from build123d import *

# Parameters (mm, degrees)
SKETCH_1_W          = 32
SKETCH_1_H          = 32
EXTRUDE_1_DEPTH     = 8
CUT_EXTRUDE_1_REACH = 10
SKETCH_2_R          = 1.5
SKETCH_3_R          = 13.25
CUT_EXTRUDE_2_DEPTH = 2.2
SKETCH_4_R          = 5.1
CUT_EXTRUDE_3_DEPTH = 3.5
CUT_EXTRUDE_4_REACH = 4.3
SKETCH_5_R          = 3
FILLET_1_R          = 2


with BuildPart() as part:
    # 草图1 → 凸台-拉伸1 (new body)
    with BuildSketch(Plane.XY):
        Rectangle(SKETCH_1_W, SKETCH_1_H)
    extrude(amount=EXTRUDE_1_DEPTH)

    # 草图2 → 切除-拉伸1 (cut, up to next)
    with BuildSketch(Plane.XY.offset(8), mode=Mode.PRIVATE) as cut_extrude_1_sk1:
        with Locations((-13.258252147, 13.258252147)):
            Circle(SKETCH_2_R)
    cut_extrude_1_tool1 = extrude(cut_extrude_1_sk1.sketch, amount=-CUT_EXTRUDE_1_REACH, mode=Mode.PRIVATE) & part.part
    add(cut_extrude_1_tool1.solids().sort_by_distance((-13.258252, 13.258252, 8))[0], mode=Mode.SUBTRACT)
    # 草图2 → 切除-拉伸1 (cut, up to next)
    with BuildSketch(Plane.XY.offset(8), mode=Mode.PRIVATE) as cut_extrude_1_sk2:
        with Locations((13.258252147, 13.258252147)):
            Circle(SKETCH_2_R)
    cut_extrude_1_tool2 = extrude(cut_extrude_1_sk2.sketch, amount=-CUT_EXTRUDE_1_REACH, mode=Mode.PRIVATE) & part.part
    add(cut_extrude_1_tool2.solids().sort_by_distance((13.258252, 13.258252, 8))[0], mode=Mode.SUBTRACT)
    # 草图2 → 切除-拉伸1 (cut, up to next)
    with BuildSketch(Plane.XY.offset(8), mode=Mode.PRIVATE) as cut_extrude_1_sk3:
        with Locations((13.258252147, -13.258252147)):
            Circle(SKETCH_2_R)
    cut_extrude_1_tool3 = extrude(cut_extrude_1_sk3.sketch, amount=-CUT_EXTRUDE_1_REACH, mode=Mode.PRIVATE) & part.part
    add(cut_extrude_1_tool3.solids().sort_by_distance((13.258252, -13.258252, 8))[0], mode=Mode.SUBTRACT)
    # 草图2 → 切除-拉伸1 (cut, up to next)
    with BuildSketch(Plane.XY.offset(8), mode=Mode.PRIVATE) as cut_extrude_1_sk4:
        with Locations((-13.258252147, -13.258252147)):
            Circle(SKETCH_2_R)
    cut_extrude_1_tool4 = extrude(cut_extrude_1_sk4.sketch, amount=-CUT_EXTRUDE_1_REACH, mode=Mode.PRIVATE) & part.part
    add(cut_extrude_1_tool4.solids().sort_by_distance((-13.258252, -13.258252, 8))[0], mode=Mode.SUBTRACT)

    # 草图3 → 切除-拉伸2 (cut)
    with BuildSketch(Plane.XY.offset(8)):
        Circle(SKETCH_3_R)
    extrude(amount=-CUT_EXTRUDE_2_DEPTH, mode=Mode.SUBTRACT)

    # 草图4 → 切除-拉伸3 (cut)
    with BuildSketch(Plane.XY.offset(5.8)):
        Circle(SKETCH_4_R)
    extrude(amount=-CUT_EXTRUDE_3_DEPTH, mode=Mode.SUBTRACT)

    # 草图5 → 切除-拉伸4 (cut, up to next)
    with BuildSketch(Plane.XY.offset(2.3), mode=Mode.PRIVATE) as cut_extrude_4_sk1:
        Circle(SKETCH_5_R)
    cut_extrude_4_tool1 = extrude(cut_extrude_4_sk1.sketch, amount=-CUT_EXTRUDE_4_REACH, mode=Mode.PRIVATE) & part.part
    add(cut_extrude_4_tool1.solids().sort_by_distance((0, 0, 2.3))[0], mode=Mode.SUBTRACT)

    # 圆角1
    fillet_1_edges = [part.edges().sort_by_distance(p)[0] for p in [
        (16, -16, 4),
        (-16, -16, 4),
        (-16, 16, 4),
        (16, 16, 4),
    ]]
    fillet(fillet_1_edges, radius=FILLET_1_R)


solid = part.part
For this review, take the finished solid that the model builds, in its own axes (mm). A direction names the side the tool comes from. Give positions to 0.01 mm unless a question says otherwise; leave off trailing zeros. Loops run counter-clockwise (first coordinate to the right, second up) from the corner with the lowest first, then second, coordinate; pieces in that order, holes last.
Item 1: Draft analysis for pull direction X (two halves, no side actions). For faces 1 (the cylindrical face through (-14.757, -13.192, 4.056)), 2 (the cylindrical face through (-15.43, -15.4, 4.06)), 3 (the cylindrical face through (15.4, 15.43, 4.06)), state which applies: +X half, -X half, draft (parallel to the pull), parting line (faces both ways), or undercut.
Item 2: Take a section at C-C, the plane z = 7. State the section outline as (x, y) points, and give its area (3 significant figures).
Item 3: Take a section at D-D, the plane y = 8. State the section outline as (x, z) points, and give its area (3 significant figures).
Item 4: For line 1 along Y through (x, z) = (0, 1.6); line 2 along Y through (x, z) = (14, 6.5); line 3 along X through (y, z) = (12.5, 5.5), list the stretches that pass through material, from the lowest coordinate up.
Item 5: Tool access review of faces 4 (the flat face through (16, 0, 4)), 5 (the cylindrical face through (7.123, 11.172, 6.915)): name each direction out of +Z, -Z, +X, -X, +Y, -Y from which nothing blocks a thin tool from reaching the whole face with its end or side.
Item 6: Insertion check: pin 1 (9 mm diameter, centred on x = 0, y = 0, fed in from +Z); pin 2 (5 mm diameter, centred on x = 1, y = -2.5, fed in from +Z); pin 3 (2.5 mm diameter, centred on x = -13.26, y = -13.26, fed in from +Z). Each pin has a flat end and moves straight along its axis. Give the tip position at first contact, or say it passes through.
Item 7: Take a section at A-A, the plane x = 0. State the section outline as (y, z) points.
Calculated:
1. face 1: undercut
1. face 2: -X half
1. face 3: +X half
2. outline: (-16, -14) arc R2 ccw to (-14, -16) - (14, -16) arc R2 ccw to (16, -14) - (16, 14) arc R2 ccw to (14, 16) - (-14, 16) arc R2 ccw to (-16, 14) - close; hole circle Ø3 at (-13.26, -13.26); hole circle Ø3 at (-13.26, 13.26); hole circle Ø26.5 at (0, 0); hole circle Ø3 at (13.26, -13.26); hole circle Ø3 at (13.26, 13.26)
2. area: 441 mm2
3. outline: (-16, 0) - (16, 0) - (16, 8) - (10.56, 8) - (10.56, 5.8) - (-10.56, 5.8) - (-10.56, 8) - (-16, 8) - close
3. area: 210 mm2
4. line 1: y = -16 to -3, 3 to 16
4. line 2: y = -16 to -14.56, -11.95 to 11.95, 14.56 to 16
4. line 3: x = -16 to -14.55, -11.96 to 11.96, 14.55 to 16
5. face 4: +Z, -Z, +X, +Y, -Y
5. face 5: +Z
6. pin 1: stops at z = 2.3
6. pin 2: stops at z = 5.8
6. pin 3: passes through
7. outline: (-16, 0) - (-3, 0) - (-3, 2.3) - (-5.1, 2.3) - (-5.1, 5.8) - (-13.25, 5.8) - (-13.25, 8) - (-16, 8) - close; (3, 0) - (16, 0) - (16, 8) - (13.25, 8) - (13.25, 5.8) - (5.1, 5.8) - (5.1, 2.3) - (3, 2.3) - close
